Source: CAD feature listing. Evaluate the final solid. Frame: model axes, mm. Face numbers are marked on the shaded views. A direction names the side the tool comes from. Round coordinates to 2 decimals unless told otherwise and drop trailing zeros. Loops run counter-clockwise (first coordinate to the right, second up) from the corner with the lowest first, then second, coordinate; pieces in that order, holes last.
(1) First-contact query: pin 1 Ø6.5 at (x, z) = (0.5, -20) entering from +Y; pin 2 Ø6 at (y, z) = (11, -3) entering from -X; pin 3 Ø3.5 at (y, z) = (6.35, 20) entering from -X; pin 4 Ø4 at (x, y) = (-9.5, 7.5) entering from -Z. Flat tips, straight axial feed; report the tip coordinate or a pass-through.
(2) Section B-B, the plane x = 0. Return the cut outline in (y, z) (3 decimals).
(3) Section A-A, the plane y = 6.35. Return the cut outline in (x, z) (3 decimals), plus the area to 3 significant figures.
(4) Section D-D, the plane x = 5.25. Return the cut outline in (y, z).
(5) Section C-C, the plane z = -20. Return the cut outline in (x, y) (3 decimals).
(6) Material intervals for probe 1 along Z at (x, y) = (-7.25, 6.35); probe 2 along Z at (x, y) = (0, 10.15); probe 3 along X at (y, z) = (10.65, -20), sorted ascending.
(7) Set-up query: the marked faces 1 and 2. Return all of +Z, -Z, +X, -X, +Y, -Y with unobstructed straight access to the full face (end or side cutting, diameter ignored); none if empty.
```python
from build123d import *

# Parameters (mm, degrees)
SKETCH2_W                     = 12.7
SKETCH2_H                     = 84
BOSS_EXTRUDE1_DEPTH           = 12.7
CBORE_FOR_M4_SHCS1_AT_2_COUNT = 2
CBORE_FOR_M4_SHCS1_AT_2_PITCH = 15
SKETCH8_W                     = 29
SKETCH8_H                     = 12.7
BOSS_EXTRUDE3_DEPTH           = 5
CBORE_FOR_M5_SHCS2_AT_2_COUNT = 2
CBORE_FOR_M5_SHCS2_AT_2_PITCH = 15


with BuildPart() as part:
    # Sketch2 → Boss-Extrude1 (new body)
    with BuildSketch(Plane(origin=(0, 0, 0), x_dir=(1, 0, 0), z_dir=(0, 1, 0))):
        Rectangle(SKETCH2_W, SKETCH2_H)
    extrude(amount=BOSS_EXTRUDE1_DEPTH)

    # Sketch4 → CBORE for M4 SHCS1 (revolve, cut)
    with BuildSketch(Plane(origin=(0, 12.7, -35), x_dir=(0, 0, 1), z_dir=(1, 0, 0))):
        Polygon((0, 0), (0, 12.7), (2.4, 12.7), (2.4, 4), (4, 4), (4, 0.020977491), (4.025, 0), align=None)
    cbore_for_m4_shcs1 = revolve(axis=Axis((0, 19.05, -35), (0, -1, 0)), mode=Mode.SUBTRACT)

    # CBORE for M4 SHCS1 at 2: CBORE for M4 SHCS1 ×2
    with Locations(*[(0, 0, i * CBORE_FOR_M4_SHCS1_AT_2_PITCH) for i in range(1, CBORE_FOR_M4_SHCS1_AT_2_COUNT)]):
        add(cbore_for_m4_shcs1, mode=Mode.SUBTRACT)

    # Sketch8 → Boss-Extrude3 (add)
    with BuildSketch(Plane.ZY.offset(6.35)):
        with Locations((27.5, 6.35)):
            Rectangle(SKETCH8_W, SKETCH8_H)
    extrude(amount=BOSS_EXTRUDE3_DEPTH)

    # Sketch7 → CBORE for M5 SHCS2 (revolve, cut)
    with BuildSketch(Plane(origin=(6.35, 6.35, 35), x_dir=(0, 0, -1), z_dir=(0, 1, 0))):
        Polygon((0, 0), (0, 17.7), (2.9, 17.7), (2.9, 5), (5, 5), (5, 0.020977491), (5.025, 0), align=None)
    cbore_for_m5_shcs2 = revolve(axis=Axis((12.7, 6.35, 35), (-1, 0, 0)), mode=Mode.SUBTRACT)

    # CBORE for M5 SHCS2 at 2: CBORE for M5 SHCS2 ×2
    with Locations(*[(0, 0, -i * CBORE_FOR_M5_SHCS2_AT_2_PITCH) for i in range(1, CBORE_FOR_M5_SHCS2_AT_2_COUNT)]):
        add(cbore_for_m5_shcs2, mode=Mode.SUBTRACT)


solid = part.part
```
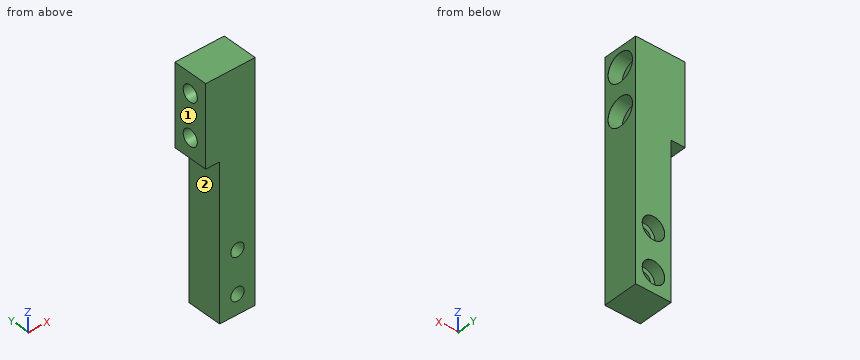
Output values:
1. pin 1: stops at y = 8.7
1. pin 2: stops at x = -6.35
1. pin 3: passes through
1. pin 4: stops at z = 13
2. outline: (0, -42) - (12.7, -42) - (12.7, -39.025) - (12.679, -39) - (8.7, -39) - (8.7, -37.4) - (0, -37.4) - close; (0, -32.6) - (8.7, -32.6) - (8.7, -31) - (12.679, -31) - (12.7, -30.975) - (12.7, -24.025) - (12.679, -24) - (8.7, -24) - (8.7, -22.4) - (0, -22.4) - close; (0, -17.6) - (8.7, -17.6) - (8.7, -16) - (12.679, -16) - (12.7, -15.975) - (12.7, 42) - (0, 42) - close; hole circle Ø5.8 at (6.35, 20); hole circle Ø5.8 at (6.35, 35)
3. outline: (-11.35, 13) - (-6.35, 13) - (-6.35, -42) - (6.35, -42) - (6.35, 14.975) - (6.329, 15) - (1.35, 15) - (1.35, 17.1) - (-11.35, 17.1) - close; (-11.35, 22.9) - (1.35, 22.9) - (1.35, 25) - (6.329, 25) - (6.35, 25.025) - (6.35, 29.975) - (6.329, 30) - (1.35, 30) - (1.35, 32.1) - (-11.35, 32.1) - close; (-11.35, 37.9) - (1.35, 37.9) - (1.35, 40) - (6.329, 40) - (6.35, 40.025) - (6.35, 42) - (-11.35, 42) - close; hole circle Ø4.8 at (0, -35); hole circle Ø4.8 at (0, -20)
3. area: 928 mm2
4. outline: (0, -42) - (12.7, -42) - (12.7, 42) - (0, 42) - close; hole circle Ø10 at (6.35, 20); hole circle Ø10 at (6.35, 35)
5. outline: (-6.35, 0) - (-2.4, 0) - (-2.4, 8.7) - (-4, 8.7) - (-4, 12.679) - (-4.025, 12.7) - (-6.35, 12.7) - close; (2.4, 0) - (6.35, 0) - (6.35, 12.7) - (4.025, 12.7) - (4, 12.679) - (4, 8.7) - (2.4, 8.7) - close
6. probe 1: z = 13 to 17.1, 22.9 to 32.1, 37.9 to 42
6. probe 2: z = -42 to -39, -31 to -24, -16 to 42
6. probe 3: x = -6.35 to -4, 4 to 6.35
7. face 1: +Z, -Z, -X, +Y, -Y
7. face 2: -Z, -X, +Y, -Y
